Can you work these out from the drawing? Everything is in mm from the part's minimum corner. A direction names the side the tool comes from. Coordinates: 2 decimals unless noted, no trailing zeros. Order: outer loops, then holes, each group sorted by start corner. A loop starts at its lowest first (then second) coordinate and runs counter-clockwise, first axis right, second up. Notation, with made-up numbers: (-2, 82.25) - (21, 82.25) arc R14 cw to (21, 104.25) - close; hole circle Ø6 at (-0.5, 51.5). An arc over 180 degrees is marked (long way). One line per item, written item: value.
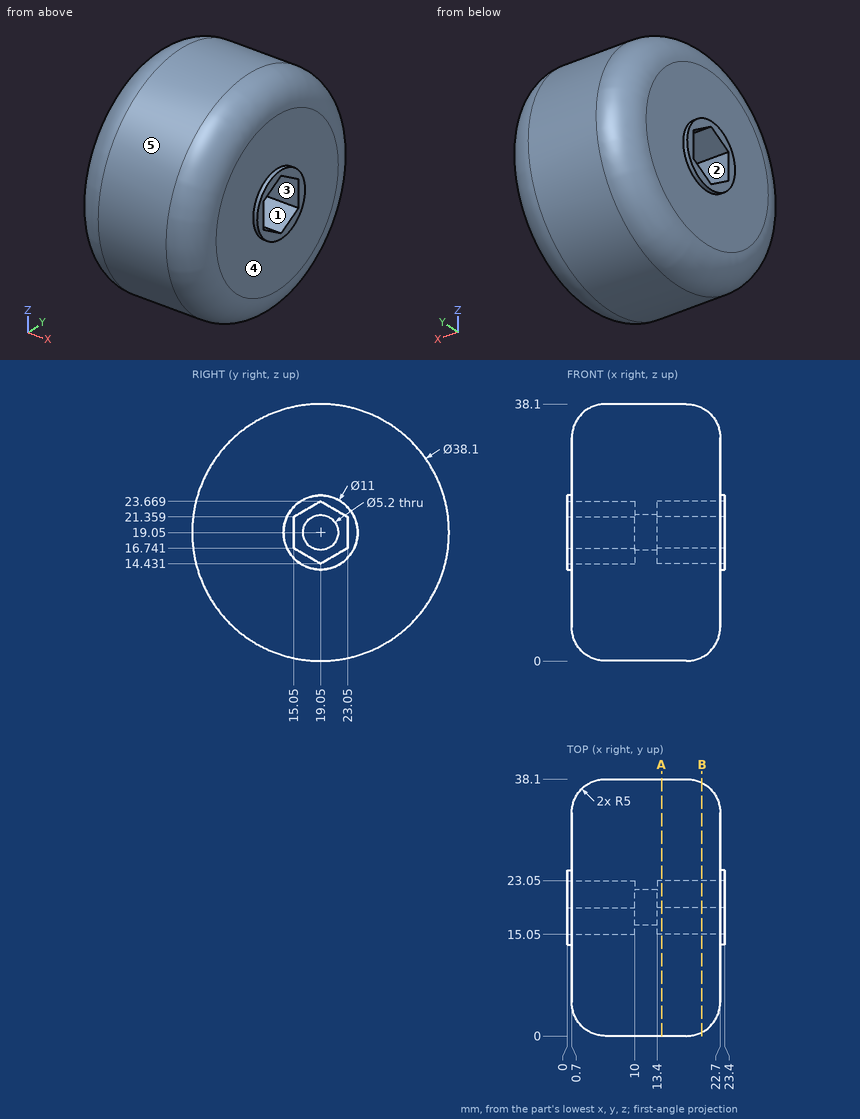
Item 1: I want a section at A-A on x = 14. Please give me the cut outline in (y, z).
Conclusion:
outline: circle Ø38.1 at (19.05, 19.05); hole (15.05, 16.74) - (19.05, 14.43) - (23.05, 16.74) - (23.05, 21.36) - (19.05, 23.67) - (15.05, 21.36) - close
Item 2: For the marked faces 1 and 2, which set-ups out of +Z, -Z, +X, -X, +Y, -Y let a thin tool reach every point of the face, with its end or its side?
Conclusion:
face 1: +X
face 2: -X
Item 3: I want a section at B-B on x = 20. Please give me the cut outline in (y, z), then the cut area to 3 significant figures.
Conclusion:
outline: circle Ø36.98 at (19.05, 19.05); hole (15.05, 16.74) - (19.05, 14.43) - (23.05, 16.74) - (23.05, 21.36) - (19.05, 23.67) - (15.05, 21.36) - close
area: 1,020 mm²
Item 4: Thinking about a two-plate mould opening in Z: for the marked faces 3, 4 and 5, which applies, pulls with the +Z half, pulls with the -Z half, needs draft (parallel to the pull), parting line crosses it, or undercut?
Conclusion:
face 3: undercut
face 4: needs draft
face 5: parting line crosses it
Item 5: I'm going to push flat-ended pins straight in: pin 1 Ø2 at (x, y) = (9, 20.5) entering from -Z (1 decimal); pin 2 Ø6 at (y, z) = (19.05, 19.05) entering from -X; pin 3 Ø2 at (x, y) = (2.5, 7) entering from -Z. Where does each tip first touch, or does it pass through?
Conclusion:
pin 1: z = 0
pin 2: x = 10
pin 3: z = 4.58
Item 6: If I drill on probe 1 along Z at (x, y) = (12.6, 19.05); probe 2 along X at (y, z) = (25, 11); probe 3 along Y at (x, z) = (6, 15.5) (1 decimal), over which ranges is the centre line in solid material (lowest first)?
Conclusion:
probe 1: 0 to 16.45, 21.65 to 38.1
probe 2: 0.7 to 22.7
probe 3: 0.3 to 17.2, 20.9 to 37.8
